Could you check a few things on this drawing? It's one solid part, dimensions in mm from its lowest x, y, z. A direction names the side the tool comes from. Give positions to 0.01 mm unless a question says otherwise; leave off trailing zeros. Order: outer loops, then holes, each group sorted by start corner. A loop starts at its lowest first (then second) coordinate and runs counter-clockwise, first axis right, second up. Notation, with made-up numbers: (-3.75, 70) -> (40.25, 70) arc R28 ccw to (40.25, 88) -> close; hole circle Ø4 at (20, -3.75). An arc over 180 degrees is marked (long way). Answer as a JSON object with one key per item and string values.
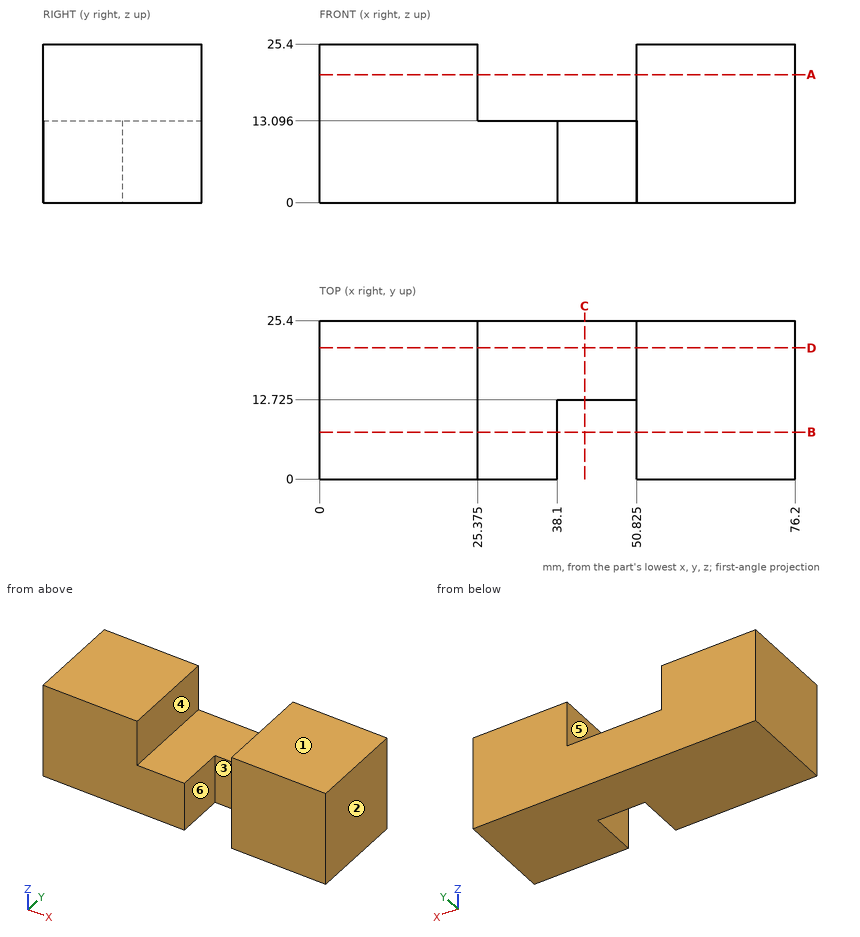
1. If we section it at C-C on x = 42.5: Please give me the cut outline in (y, z) (1 decimal).
Worked answers:
{"outline": "(12.7, 0) -> (25.4, 0) -> (25.4, 13.1) -> (12.7, 13.1) -> close"}
2. If we section it at B-B on y = 7.5: Please give me the cut outline in (x, z) (1 decimal), then the cut area to 3 significant figures.
Worked answers:
{"outline": "(0, 0) -> (38.1, 0) -> (38.1, 13.1) -> (25.4, 13.1) -> (25.4, 25.4) -> (0, 25.4) -> close; (50.8, 0) -> (76.2, 0) -> (76.2, 25.4) -> (50.8, 25.4) -> close", "area": "1,460 mm²"}
3. If we section it at A-A on z = 20.5: Please give me the cut outline in (x, y) (1 decimal).
Worked answers:
{"outline": "(0, 0) -> (25.4, 0) -> (25.4, 25.4) -> (0, 25.4) -> close; (50.8, 0) -> (76.2, 0) -> (76.2, 25.4) -> (50.8, 25.4) -> close"}
4. Please list where these lines run through material, in increasing order: L1, parallel to X at y = 12.75, z = 18.25 (1 decimal); L2, parallel to X at y = 11.25, z = 7 (1 decimal); L3, parallel to Z at x = 34.5, y = 7.5 (1 decimal).
Worked answers:
{"L1": "0 to 25.4, 50.8 to 76.2", "L2": "0 to 38.1, 50.8 to 76.2", "L3": "0 to 13.1"}
5. Will this pin go through, and if not, where does the flat tip stop? pin 1 Ø12.5 at (x, y) = (42, 13.5) entering from +Z.
Worked answers:
{"pin 1": "z = 13.1"}
6. If we section it at D-D on y = 21: Please give me the cut outline in (x, z) (1 decimal).
Worked answers:
{"outline": "(0, 0) -> (76.2, 0) -> (76.2, 25.4) -> (50.8, 25.4) -> (50.8, 13.1) -> (25.4, 13.1) -> (25.4, 25.4) -> (0, 25.4) -> close"}
7. For the marked faces 4, 5 and 6, which set-ups out of +Z, -Z, +X, -X, +Y, -Y let a thin tool reach every point of the face, with its end or its side?
Worked answers:
{"face 4": "+Z, +Y, -Y", "face 5": "+Z, -Y", "face 6": "+Z, -Z, -Y"}
8. If we mould it in two halves opening along X, with no side actions, what happens to the marked faces 1, 2 and 3? For each: +X half, -X half, draft (parallel to the pull), parting line (faces both ways), or undercut.
Worked answers:
{"face 1": "draft", "face 2": "+X half", "face 3": "undercut"}
